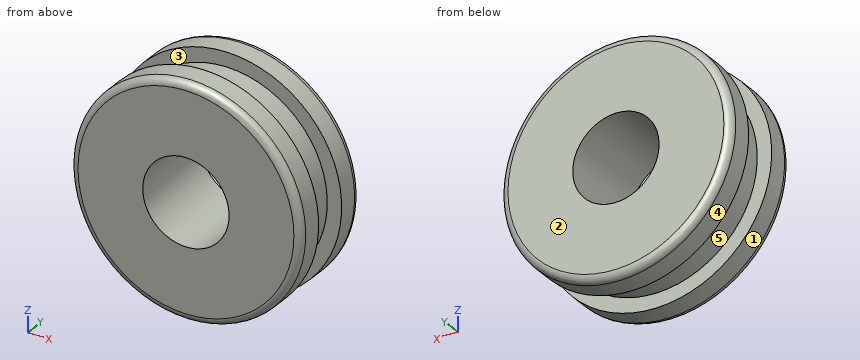
```python
from build123d import *

# Parameters (mm, degrees)
CROQUIS_BASE_R           = 3.5
SALIENTE_EXTRUIR3_DEPTH  = 1.25
CROQUIS_CAP_R            = 4
SALIENTE_EXTRUIR4_DEPTH  = 0.95
REDONDEO1_R              = 0.25
REDONDEO1_OF_SIMETR_A1_R = 0.25
CROQUIS_BARRENO_R        = 1.5
CORTAR_EXTRUIR1_DEPTH    = 7.474758683


with BuildPart() as part:
    # Croquis base → Saliente-Extruir3 (new body)
    with BuildSketch(Plane(origin=(0, 0, 0), x_dir=(1, 0, 0), z_dir=(0, 1, 0))):
        with Locations(Location((0, 0, 0), (0, 0, 270))):
            Circle(CROQUIS_BASE_R)
    extrude(amount=SALIENTE_EXTRUIR3_DEPTH)

    # Croquis cap → Saliente-Extruir4 (add)
    with BuildSketch(Plane(origin=(0, 1.25, 0), x_dir=(1, 0, 0), z_dir=(0, 1, 0))):
        with Locations(Location((0, 0, 0), (0, 0, 90))):
            Circle(CROQUIS_CAP_R)
    saliente_extruir4 = extrude(amount=SALIENTE_EXTRUIR4_DEPTH)

    # Redondeo1
    redondeo1_edges = [part.edges().sort_by_distance(p)[0] for p in [
        (0, 2.2, 4),
    ]]
    fillet(redondeo1_edges, radius=REDONDEO1_R)

    # Simetría1: Saliente-Extruir4 across plane
    add(saliente_extruir4.mirror(Plane.ZX.offset(0.625)))

    # Redondeo1 of Simetría1
    redondeo1_of_simetr_a1_edges = [part.edges().sort_by_distance(p)[0] for p in [
        (0, -0.95, 4),
    ]]
    fillet(redondeo1_of_simetr_a1_edges, radius=REDONDEO1_OF_SIMETR_A1_R)

    # Croquis barreno → Cortar-Extruir1 (cut, through all)
    with BuildSketch(Plane(origin=(0, 2.2, 0), x_dir=(1, 0, 0), z_dir=(0, 1, 0))):
        with Locations(Location((0, 0, 0), (0, 0, 270))):
            Circle(CROQUIS_BARRENO_R)
    extrude(amount=-CORTAR_EXTRUIR1_DEPTH, mode=Mode.SUBTRACT)


solid = part.part
```
Design review of the part built by this model. Coordinates are the model's own, in mm. Face numbers are marked on the shaded views. A direction names the side the tool comes from. Round coordinates to 2 decimals unless told otherwise and drop trailing zeros. Order: outer loops, then holes, each group sorted by start corner. A loop starts at its lowest first (then second) coordinate and runs counter-clockwise, first axis right, second up. Notation, with made-up numbers: M 73.25,-11.75 L 107.25,-11.75 A32 ccw 107.25,16.25 Z; hole C -28,-2 d9. An arc over 180 degrees is marked long. Put each result on its own line as item: value.
Q1. To check wall thickness, follow line 1 (X direction, y = 1, z = 0); line 2 (X direction, y = -0.1, z = 0); line 3 (Y direction, x = -3.5, z = 1.5). State the ranges of each line that lie inside material, in increasing order.
Reported:
line 1: -3.5 to -1.5, 1.5 to 3.5
line 2: -4 to -1.5, 1.5 to 4
line 3: -0.94 to 0, 1.25 to 2.19
Q2. Consider section D-D (y = 1.5). State the section outline as (x, z) points, and give its area (3 significant figures).
Reported:
outline: C 0,0 d8; hole C 0,0 d3
area: 43.2 mm²
Q3. Consider section C-C (y = 0.75). State the section outline as (x, z) points.
Reported:
outline: C 0,0 d7; hole C 0,0 d3
Q4. Machinability: for the marked faces 4 and 5, which of the approach directions +Z, -Z, +X, -X, +Y, -Y give a long, thin tool a straight path to every point of the face, cutting with its end or side? Answer none if there is none.
Reported:
face 4: +Y, -Y
face 5: none
Q5. Consider section B-B (x = 0). State the section outline as (y, z) points.
Reported:
outline: M -0.95,-3.75 A0.25 ccw -0.7,-4 L 0,-4 L 0,-3.5 L 1.25,-3.5 L 1.25,-4 L 1.95,-4 A0.25 ccw 2.2,-3.75 L 2.2,-1.5 L -0.95,-1.5 Z; M -0.95,1.5 L 2.2,1.5 L 2.2,3.75 A0.25 ccw 1.95,4 L 1.25,4 L 1.25,3.5 L 0,3.5 L 0,4 L -0.7,4 A0.25 ccw -0.95,3.75 Z
Q6. Insertion check: pin 1 Ø1 at (x, z) = (-0.5, 0) entering from -Y; pin 2 Ø1 at (x, y) = (-1.5, 1) entering from -Z. Each pin has a flat end and moves straight along its axis. Give the tip position at first contact, or say it passes through.
Reported:
pin 1: through
pin 2: z = -3.86
Q7. Draft analysis for pull direction Y (two halves, no side actions). For the marked faces 1, 2 and 3, state which applies: released by +Y, released by -Y, zero draft, split by the parting line, or undercut.
Reported:
face 1: zero draft
face 2: released by +Y
face 3: undercut
Q8. Consider section A-A (z = 0). State the section outline as (x, y) points.
Reported:
outline: M -4,-0.7 A0.25 ccw -3.75,-0.95 L -1.5,-0.95 L -1.5,2.2 L -3.75,2.2 A0.25 ccw -4,1.95 L -4,1.25 L -3.5,1.25 L -3.5,0 L -4,0 Z; M 1.5,-0.95 L 3.75,-0.95 A0.25 ccw 4,-0.7 L 4,0 L 3.5,0 L 3.5,1.25 L 4,1.25 L 4,1.95 A0.25 ccw 3.75,2.2 L 1.5,2.2 Z
